from build123d import *

# Parameters (mm, degrees)
F0_W      = 25.4
F0_H      = 25.4
F1_DEPTH  = 29.464
F1_TAPER  = 34
F1_FACE_W = 25.4
F1_FACE_H = 25.4


# Not quite as in the source:
# - an extrude whose draft closes it to a point is written as a loft to that point


with BuildPart() as f1:
    # F0 (on Top) → F1 (new body)
    with BuildSketch(Plane.XY):
        Rectangle(F0_W, F0_H)
    extrude(amount=F1_DEPTH, taper=F1_TAPER)

    # F1_face (on face) → F2 section 0
    with BuildSketch(Plane(origin=(0, 0, 0), x_dir=(1, 0, 0), z_dir=(0, 0, -1)), mode=Mode.PRIVATE) as f2_s0:
        Rectangle(F1_FACE_W, F1_FACE_H)
    loft([f2_s0.sketch, Vertex(0, 0, -18.8285243001)], ruled=True)


solid = f1.part
The listing builds one solid part. Answer for the finished solid, in the listing's coordinates (mm). Give positions to 0.01 mm unless a question says otherwise; leave off trailing zeros. Write each loop counter-clockwise with the first axis right and the second up, starting at its lowest first coordinate (ties: lowest second). Pieces come first, ordered by that corner, then holes.
1) Section C-C (z = -2.5) is taken. Write down the section's boundary in (x, y), and give its area (3 significant figures).
2) Given P1, Ø12, axis at x = -2, z = 6.5, coming from the -Y side; P2, Ø12, axis at y = -4.5, z = -13.5, coming from the +X side; P3, Ø5, axis at x = 4, z = 8, coming from the -Y side, each flat-ended and moving along its own axis, determine where each tip first touches the part or whether it passes through.
3) Section D-D (z = 8) is taken. Write down the section's boundary in (x, y).
4) Find the intervals of material crossed by L1, parallel to X at y = 4.25, z = -5.5; L2, parallel to X at y = -8.5, z = 4.5; L3, parallel to Z at x = -10, y = -9.25, in increasing order.
5) Section B-B (y = -5.5) is taken. Write down the section's boundary in (x, z), and give its area (3 significant figures).
6) Section A-A (x = 8) is taken. Write down the section's boundary in (y, z), and give its area (3 significant figures).
Response:
1. outline: (-11.01, -11.01) - (11.01, -11.01) - (11.01, 11.01) - (-11.01, 11.01) - close
1. area: 485 mm2
2. P1: stops at y = -12.36
2. P2: stops at x = 7.64
2. P3: stops at y = -8.99
3. outline: (-7.3, -7.3) - (7.3, -7.3) - (7.3, 7.3) - (-7.3, 7.3) - close
4. L1: x = -8.99 to 8.99
4. L2: x = -9.66 to 9.66
4. L3: z = -4 to 4
5. outline: (-12.7, 0) - (-5.5, -10.67) - (5.5, -10.67) - (12.7, 0) - (5.5, 10.67) - (-5.5, 10.67) - close
5. area: 389 mm2
6. outline: (-12.7, 0) - (-8, -6.97) - (8, -6.97) - (12.7, 0) - (8, 6.97) - (-8, 6.97) - close
6. area: 288 mm2
